Check sheet for the modelled part. Datum: model origin and axes. Units: mm. Round coordinates to 2 decimals unless told otherwise and drop trailing zeros. Order: outer loops, then holes, each group sorted by start corner. A loop starts at its lowest first (then second) coordinate and runs counter-clockwise, first axis right, second up. Notation, with made-up numbers: (42.5, 73.5) -> (91.5, 73.5) arc R28 cw to (91.5, 101.5) -> close; hole circle Ø6 at (-12.75, 78.5). An arc over 180 degrees is marked (long way). Answer in a Markdown table with one row per item.
from build123d import *

# Parameters (mm, degrees)
F0_W     = 152.4
F0_H     = 152.4
F0_R     = 6.35
F1_DEPTH = 25.4
F2_D     = 4.2


with BuildPart() as f1:
    # F0 (on Top) → F1 (new body)
    with BuildSketch(Plane.XY):
        Rectangle(F0_W, F0_H)
        Circle(F0_R, mode=Mode.SUBTRACT)
    extrude(amount=-F1_DEPTH)

    # F2 (through all)
    with Locations(Plane.XY):
        with Locations((0, 65.0875), (-56.3674284688, 32.54375), (-56.3674284688, -32.54375), (0, -65.0875), (56.3674284688, -32.54375), (56.3674284688, 32.54375)):
            Hole(F2_D / 2)


solid = f1.part
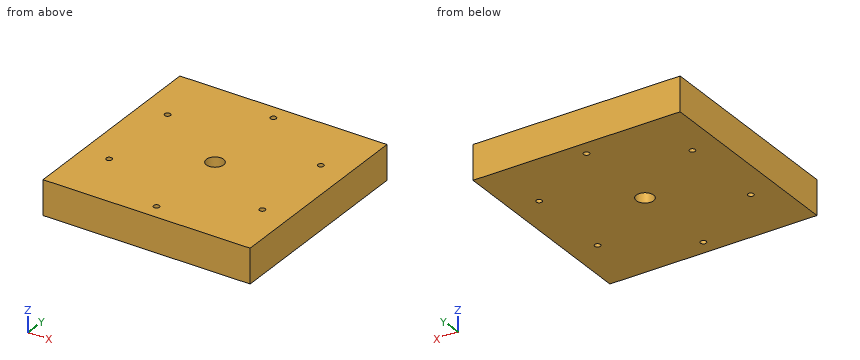
Item 1: Cross-section at B-B (y = 0). Record the boundary of the cut face in (x, z), and give its area (3 significant figures).
Result sheet:
| item | result |
|---|---|
| outline | (-76.2, -25.4) -> (-6.35, -25.4) -> (-6.35, 0) -> (-76.2, 0) -> close; (6.35, -25.4) -> (76.2, -25.4) -> (76.2, 0) -> (6.35, 0) -> close |
| area | 3,550 mm^2 |
Item 2: Cross-section at A-A (x = 0). Record the boundary of the cut face in (y, z).
Result sheet:
| item | result |
|---|---|
| outline | (-76.2, -25.4) -> (-67.19, -25.4) -> (-67.19, 0) -> (-76.2, 0) -> close; (-62.99, -25.4) -> (-6.35, -25.4) -> (-6.35, 0) -> (-62.99, 0) -> close; (6.35, -25.4) -> (62.99, -25.4) -> (62.99, 0) -> (6.35, 0) -> close; (67.19, -25.4) -> (76.2, -25.4) -> (76.2, 0) -> (67.19, 0) -> close |
Item 3: Depth check by flat-ended pin: P1, Ø4, axis at x = -56.37, y = -32.54, coming from the +Z side. Enter the tip coordinate at first touch or a pass-through.
Result sheet:
| item | result |
|---|---|
| P1 | passes through |
Item 4: Scan lines: line 1 (Y direction, x = 0, z = -11.25); line 2 (X direction, y = -34, z = -22.75); line 3 (X direction, y = -31, z = -5.75). Record each from-to range of solid material in increasing order. Write a range as [from, to].
Result sheet:
| item | result |
|---|---|
| line 1 | y = [-76.2, -67.19], [-62.99, -6.35], [6.35, 62.99], [67.19, 76.2] |
| line 2 | x = [-76.2, -57.88], [-54.85, 54.85], [57.88, 76.2] |
| line 3 | x = [-76.2, -57.79], [-54.94, 54.94], [57.79, 76.2] |
